Build history of the part. All positions in model axes, mm. Face numbers are marked on the shaded views. A direction names the side the tool comes from. Give positions to 0.01 mm unless a question says otherwise; leave off trailing zeros. Write each loop counter-clockwise with the first axis right and the second up, starting at its lowest first coordinate (ties: lowest second). Pieces come first, ordered by that corner, then holes.
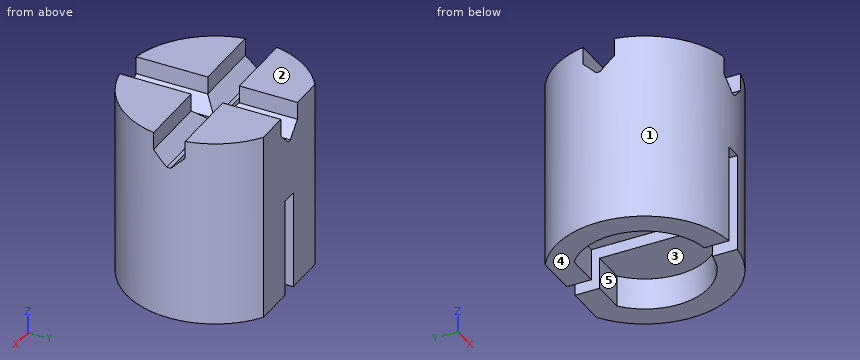
from build123d import *

# Parameters (mm, degrees)
PAD_DEPTH       = 1.6
PAD019_DEPTH    = 8
POCKET018_DEPTH = 1.6
CHAMFER_SIZE    = 0.7
SKETCH034_W     = 0.8
SKETCH034_H     = 9
POCKET019_DEPTH = 5


with BuildPart() as part:
    # Sketch031 → Pad (new body)
    with BuildSketch(Plane.XY.offset(3.15)):
        with BuildLine():
            ThreePointArc((11.492531, -46.434), (13.98, -54.684), (16.467469, -46.434))
            Line((11.492531, -46.434), (16.467469, -46.434))
        make_face()
        with BuildLine():
            ThreePointArc((11.903344, -47.684), (13.98, -53.434), (16.056656, -47.684))
            Line((11.903344, -47.684), (16.056656, -47.684))
        make_face(mode=Mode.SUBTRACT)
    extrude(amount=-PAD_DEPTH)

    # Sketch032 → Pad019 (join)
    with BuildSketch(Plane.XY.offset(3.15)):
        with BuildLine():
            ThreePointArc((11.492531, -46.434), (13.98, -54.684), (16.467469, -46.434))
            Line((11.492531, -46.434), (16.467469, -46.434))
        make_face()
    extrude(amount=PAD019_DEPTH)

    # Sketch033 → Pocket018 (cut)
    with BuildSketch(Plane.XY.offset(11.15)):
        Polygon((14.78, -54.684), (14.78, -50.984), (18.48, -50.984), (18.48, -49.384), (14.78, -49.384), (14.78, -45.684), (13.18, -45.684), (13.18, -49.384), (9.48, -49.384), (9.48, -50.984), (13.18, -50.984), (13.18, -54.684), align=None)
    extrude(amount=-POCKET018_DEPTH, mode=Mode.SUBTRACT)

    # Chamfer
    chamfer_edges = [part.edges().sort_by_distance(p)[0] for p in [
        (16.594159, -50.984, 9.55),
        (14.78, -47.909, 9.55),
        (13.18, -47.909, 9.55),
        (11.365841, -50.984, 9.55),
        (11.365841, -49.384, 9.55),
        (13.18, -52.798159, 9.55),
        (16.594159, -49.384, 9.55),
        (14.78, -52.798159, 9.55),
    ]]
    chamfer(chamfer_edges, length=CHAMFER_SIZE)

    # Sketch034 → Pocket019 (cut)
    with BuildSketch(Plane(origin=(0, 0, 1.55), x_dir=(1, 0, 0), z_dir=(0, 0, -1))):
        with Locations((13.98, 50.184)):
            Rectangle(SKETCH034_W, SKETCH034_H)
    extrude(amount=-POCKET019_DEPTH, mode=Mode.SUBTRACT)


solid = part.part
1. Drop flat-ended pins along their axis: pin 1 (0.7 mm diameter, centred on y = -47.5, z = 11, fed in from -X); pin 2 (1.5 mm diameter, centred on y = -52.5, z = 5, fed in from +X); pin 3 (1 mm diameter, centred on x = 12, z = 10.5, fed in from -Y). Give the stop position or say it passes through.
2. Mould opens along X. For the marked faces 1, 2 and 3 say: pulls with the +X half, pulls with the -X half, needs draft (parallel to the pull), parting line crosses it, or undercut.
3. Saw through at A-A on y = -50.5. Give the cut face in (x, z), plus the area to 3 significant figures.
4. Saw through at D-D on x = 16.25. Give the cut face in (y, z), plus the area to 3 significant figures.
5. Saw through at B-B on x = 10.25. Give the cut face in (y, z), plus the area to 3 significant figures.
6. 3-axis set-ups, long thin cutter, end or side, ignore diameter. For the marked faces 4 and 5: which of +Z, -Z, +X, -X, +Y, -Y reach the whole face in a straight line?
7. Drill centre lines: line 1 along X through (y, z) = (-51, 4.25); line 2 along X through (y, z) = (-50, 5.5); line 3 along Y through (x, z) = (12.5, 10.75). Where is each one in solid material? Low to high.
8. Saw through at C-C on y = -52.5. Give the cut face in (x, z).
Outcome:
1. pin 1: stops at x = 10.13
1. pin 2: stops at x = 18.2
1. pin 3: stops at y = -54.43
2. face 1: parting line crosses it
2. face 2: needs draft
2. face 3: undercut
3. outline: (9.49, 1.55) - (10.75, 1.55) - (10.75, 3.15) - (13.58, 3.15) - (13.58, 6.55) - (14.38, 6.55) - (14.38, 3.15) - (17.21, 3.15) - (17.21, 1.55) - (18.47, 1.55) - (18.47, 9.77) - (14.3, 9.77) - (14.08, 9.55) - (13.88, 9.55) - (13.66, 9.77) - (9.49, 9.77) - close
3. area: 60.6 mm2
4. outline: (-54.07, 1.55) - (-52.51, 1.55) - (-52.51, 3.15) - (-47.86, 3.15) - (-47.86, 1.55) - (-46.43, 1.55) - (-46.43, 11.15) - (-49.38, 11.15) - (-49.38, 10.25) - (-50.08, 9.55) - (-50.28, 9.55) - (-50.98, 10.25) - (-50.98, 11.15) - (-54.07, 11.15) - close
4. area: 63.8 mm2
5. outline: (-52.7, 1.55) - (-47.67, 1.55) - (-47.67, 11.15) - (-49.38, 11.15) - (-49.38, 10.25) - (-50.08, 9.55) - (-50.28, 9.55) - (-50.98, 10.25) - (-50.98, 11.15) - (-52.7, 11.15) - close
5. area: 46.3 mm2
6. face 4: -Z, +X, -X, +Y, -Y
6. face 5: -Z
7. line 1: x = 9.55 to 13.58, 14.38 to 18.41
7. line 2: x = 9.48 to 13.58, 14.38 to 18.48
7. line 3: y = -54.43 to -50.98, -49.38 to -46.43
8. outline: (10.12, 1.55) - (11.7, 1.55) - (11.7, 3.15) - (13.58, 3.15) - (13.58, 6.55) - (14.38, 6.55) - (14.38, 3.15) - (16.26, 3.15) - (16.26, 1.55) - (17.84, 1.55) - (17.84, 11.15) - (14.78, 11.15) - (14.78, 10.25) - (14.08, 9.55) - (13.88, 9.55) - (13.18, 10.25) - (13.18, 11.15) - (10.12, 11.15) - close
